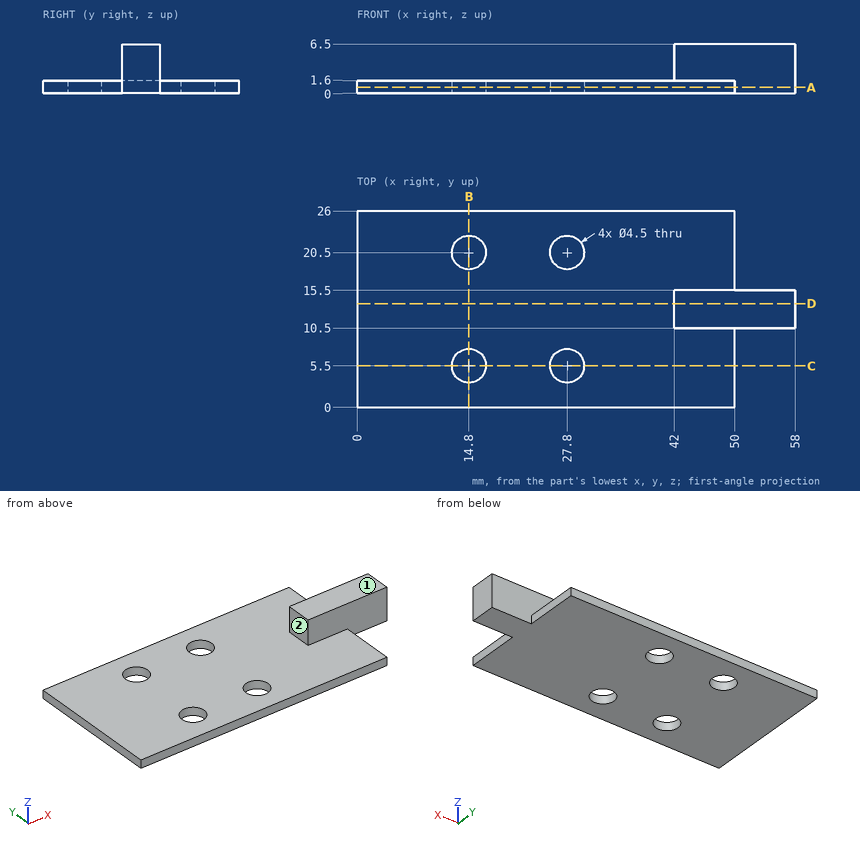
Input: dimensioned drawing with shaded views. Units: mm. Origin: part minimum x, y, z. A direction names the side the tool comes from. Round coordinates to 2 decimals unless told otherwise and drop trailing zeros. Loops run counter-clockwise (first coordinate to the right, second up) from the corner with the lowest first, then second, coordinate; pieces in that order, holes last. Notation, with made-up numbers: M 27.5,60.25 L 82.5,60.25 A13 cw 82.5,67.25 Z; hole C 57,52.25 d11. An arc over 180 degrees is marked long. Answer in a Markdown table with one row per item. Add a question column.
1. Section B-B (x = 14.8). Output: boundary loops of the cut face in (y, z), and give its area (3 significant figures).
2. Section A-A (z = 0.75). Output: boundary loops of the cut face in (x, y).
3. Section D-D (y = 13.75). Output: boundary loops of the cut face in (x, z), and give its area (3 significant figures).
4. Section C-C (y = 5.5). Output: boundary loops of the cut face in (x, z).
5. Set-up query: the marked faces 1 and 2. Return all of +Z, -Z, +X, -X, +Y, -Y with unobstructed straight access to the full face (end or side cutting, diameter ignored); none if empty.
6. Contact query for flat-ended pins moving along their axis: pin 1 (4 mm diameter, centred on x = 14.8, y = 20.5, fed in from +Z); pin 2 (7 mm diameter, centred on x = 27.8, y = 5.5, fed in from +Z); pin 3 (0.5 mm diameter, centred on y = 3, z = 1, fed in from +X); pin 4 (3 mm diameter, centred on x = 48, z = 5, fed in from +Y). Output: stop coordinate, or through.
7. Ray query, probe 1 along Y at (x, z) = (27.8, 0.75); probe 2 along X at (y, z) = (20.5, 0.85); probe 3 along X at (y, z) = (18.5, 0.5). Return the intervals inside material, ascending.
Values follow:
| question | item | result |
|---|---|---|
| 1 | outline | M 0,0 L 3.25,0 L 3.25,1.6 L 0,1.6 Z; M 7.75,0 L 18.25,0 L 18.25,1.6 L 7.75,1.6 Z; M 22.75,0 L 26,0 L 26,1.6 L 22.75,1.6 Z |
| 1 | area | 27.2 mm^2 |
| 2 | outline | M 0,0 L 50,0 L 50,10.5 L 58,10.5 L 58,15.5 L 50,15.5 L 50,26 L 0,26 Z; hole C 14.8,5.5 d4.5; hole C 14.8,20.5 d4.5; hole C 27.8,5.5 d4.5; hole C 27.8,20.5 d4.5 |
| 3 | outline | M 0,0 L 58,0 L 58,6.5 L 42,6.5 L 42,1.6 L 0,1.6 Z |
| 3 | area | 171 mm^2 |
| 4 | outline | M 0,0 L 12.55,0 L 12.55,1.6 L 0,1.6 Z; M 17.05,0 L 25.55,0 L 25.55,1.6 L 17.05,1.6 Z; M 30.05,0 L 50,0 L 50,1.6 L 30.05,1.6 Z |
| 5 | face 1 | +Z, +X, -X, +Y, -Y |
| 5 | face 2 | +Z, -X, +Y, -Y |
| 6 | pin 1 | through |
| 6 | pin 2 | z = 1.6 |
| 6 | pin 3 | x = 50 |
| 6 | pin 4 | y = 15.5 |
| 7 | probe 1 | 0 to 3.25, 7.75 to 18.25, 22.75 to 26 |
| 7 | probe 2 | 0 to 12.55, 17.05 to 25.55, 30.05 to 50 |
| 7 | probe 3 | 0 to 13.77, 15.83 to 26.77, 28.83 to 50 |
